```python
from build123d import *

# Parameters (mm, degrees)
SKETCH1_W           = 120
SKETCH1_H           = 80
SKETCH1_R           = 1.13
SKETCH1_W_2         = 3
SKETCH1_H_2         = 1.3
SKETCH1_W_3         = 1.3
SKETCH1_H_3         = 3
BOSS_EXTRUDE1_DEPTH = 8
CUT_EXTRUDE1_DEPTH  = 4
CHAMFER1_SIZE       = 1
CUT_EXTRUDE2_REACH  = 74.553
SKETCH3_W           = 20
SKETCH3_H           = 8
SKETCH4_W           = 20
SKETCH4_H           = 8
BOSS_EXTRUDE2_DEPTH = 8


with BuildPart() as part:
    # Sketch1 → Boss-Extrude1 (new body)
    with BuildSketch(Plane(origin=(0, 0, 0), x_dir=(1, 0, 0), z_dir=(0, 1, 0))):
        Rectangle(SKETCH1_W, SKETCH1_H)
        with Locations(Location((38.07, 32.68, 0), (0, 0, 270))):
            Circle(SKETCH1_R, mode=Mode.SUBTRACT)
        with Locations(Location((5.56, 17.26, 0), (0, 0, 270))):
            Circle(SKETCH1_R, mode=Mode.SUBTRACT)
        with Locations((16, -34.65)):
            Rectangle(SKETCH1_W_2, SKETCH1_H_2, mode=Mode.SUBTRACT)
        with Locations((16, -6.85)):
            Rectangle(SKETCH1_W_2, SKETCH1_H_2, mode=Mode.SUBTRACT)
        with Locations((39, -6.85)):
            Rectangle(SKETCH1_W_2, SKETCH1_H_2, mode=Mode.SUBTRACT)
        with Locations((39, -34.65)):
            Rectangle(SKETCH1_W_2, SKETCH1_H_2, mode=Mode.SUBTRACT)
        with Locations((50.65, -20.75)):
            Rectangle(SKETCH1_W_3, SKETCH1_H_3, mode=Mode.SUBTRACT)
        with Locations((4.35, -20.75)):
            Rectangle(SKETCH1_W_3, SKETCH1_H_3, mode=Mode.SUBTRACT)
        with Locations((-55.65, -20.75)):
            Rectangle(SKETCH1_W_3, SKETCH1_H_3, mode=Mode.SUBTRACT)
        with Locations((-9.35, -20.75)):
            Rectangle(SKETCH1_W_3, SKETCH1_H_3, mode=Mode.SUBTRACT)
        with Locations((-44, -34.65)):
            Rectangle(SKETCH1_W_2, SKETCH1_H_2, mode=Mode.SUBTRACT)
        with Locations((-44, -6.85)):
            Rectangle(SKETCH1_W_2, SKETCH1_H_2, mode=Mode.SUBTRACT)
        with Locations((-21, -34.65)):
            Rectangle(SKETCH1_W_2, SKETCH1_H_2, mode=Mode.SUBTRACT)
        with Locations((-21, -6.85)):
            Rectangle(SKETCH1_W_2, SKETCH1_H_2, mode=Mode.SUBTRACT)
    extrude(amount=BOSS_EXTRUDE1_DEPTH)

    # Sketch2 → Cut-Extrude1 (cut)
    with BuildSketch(Plane.XZ):
        Polygon((7.869401077, -17.26), (6.714700538, -15.26), (4.405299462, -15.26), (3.250598923, -17.26), (4.405299462, -19.26), (6.714700538, -19.26), align=None)
        Polygon((40.379401077, -32.68), (39.224700538, -30.68), (36.915299462, -30.68), (35.760598923, -32.68), (36.915299462, -34.68), (39.224700538, -34.68), align=None)
    extrude(amount=-CUT_EXTRUDE1_DEPTH, mode=Mode.SUBTRACT)

    # Chamfer1
    chamfer1_edges = [part.edges().sort_by_distance(p)[0] for p in [
        (0, 0, -40),
        (0, 0, 40),
    ]]
    chamfer(chamfer1_edges, length=CHAMFER1_SIZE)

    # Sketch3 → Cut-Extrude2 (cut, up to next)
    with BuildSketch(Plane.XZ, mode=Mode.PRIVATE) as cut_extrude2_sk1:
        with Locations((-30, 0)):
            Rectangle(SKETCH3_W, SKETCH3_H)
    cut_extrude2_tool1 = extrude(cut_extrude2_sk1.sketch, amount=-CUT_EXTRUDE2_REACH, mode=Mode.PRIVATE) & part.part
    cut_extrude2 = cut_extrude2_tool1.solids().sort_by_distance((-30, 0, 0))[0]
    add(cut_extrude2, mode=Mode.SUBTRACT)

    # Mirror1: Cut-Extrude2 across plane
    add(cut_extrude2.mirror(Plane.ZY), mode=Mode.SUBTRACT)

    # Sketch4 → Boss-Extrude2 (add)
    with BuildSketch(Plane.ZY.offset(60)):
        with Locations((20, 4)):
            Rectangle(SKETCH4_W, SKETCH4_H)
        with Locations((-20, 4)):
            Rectangle(SKETCH4_W, SKETCH4_H)
    boss_extrude2 = extrude(amount=BOSS_EXTRUDE2_DEPTH)

    # Mirror2: Boss-Extrude2 across plane
    add(boss_extrude2.mirror(Plane.ZY))


solid = part.part
```
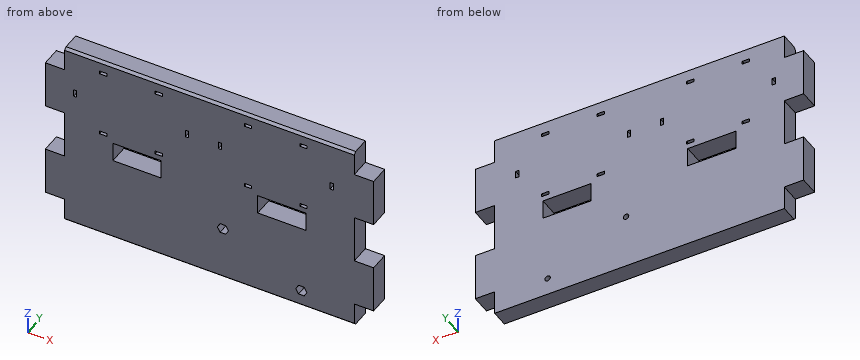
Could you check a few things on this model? Use its own coordinates, in mm. Coordinates: 2 decimals unless noted, no trailing zeros. Order: outer loops, then holes, each group sorted by start corner. A loop starts at its lowest first (then second) coordinate and runs counter-clockwise, first axis right, second up. Notation, with made-up numbers: M 30,23.25 L 39,23.25 A20 cw 39,61.25 Z; hole C 66.5,-34.5 d2. An arc over 180 degrees is marked long. Use one line per item in the form item = value. Start each with the question number.
1. For pin 1 (2.5 mm diameter, centred on x = 64.5, y = 5.5, fed in from -Z); pin 2 (1.4 mm diameter, centred on y = 5, z = 34.5, fed in from +X); pin 3 (2.5 mm diameter, centred on y = 2, z = 37, fed in from -X), each with a flat end and sliding along its axis, tell me the tip position at first contact or that it passes through.
2. Please list where these lines run through material, in increasing order: line 1 (X direction, y = 4.25, z = -2.5); line 2 (X direction, y = 4.95, z = -32.68); line 3 (X direction, y = 5.05, z = -17.26).
3. Suppose I cut it at B-B on y = 5.5. Count the separate pieces of the cut face and the enclosed holes in it, then the cut area to 3 significant figures.
4. Suppose I cut it at A-A on x = 28. Write out the boundary of the cut face in (y, z).
Geometry says:
q1.pin_1 = -30
q1.pin_2 = 60
q1.pin_3 = -60
q2.line_1 = -60 to -40, -20 to 20, 40 to 60
q2.line_2 = -60 to 36.94, 39.2 to 60
q2.line_3 = -68 to 4.43, 6.69 to 68
q3.separate_pieces = 1
q3.enclosed_holes = 16
q3.area = 9,870 mm^2
q4.outline = M 0,-39 L 1,-40 L 8,-40 L 8,-4 L 0,-4 Z; M 0,4 L 8,4 L 8,40 L 1,40 L 0,39 Z
